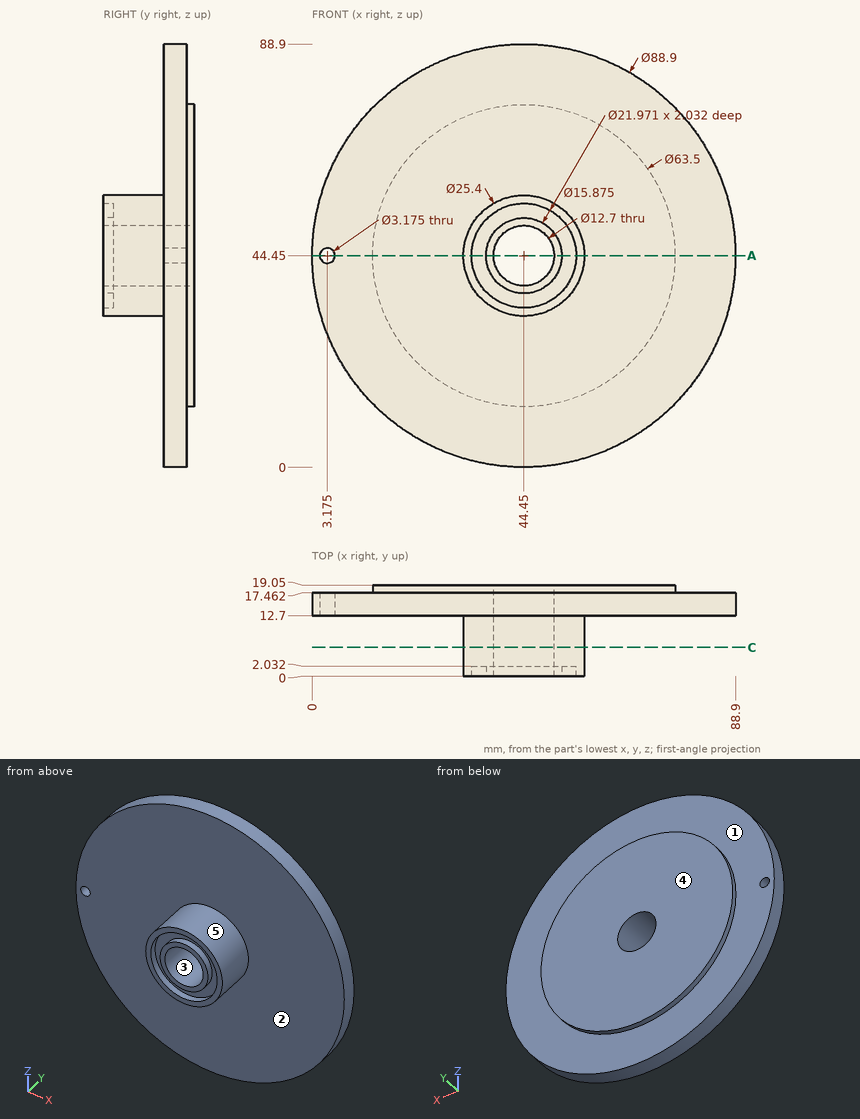
Could you check a few things on this drawing? It's one solid part, dimensions in mm from its lowest x, y, z. A direction names the side the tool comes from. Coordinates: 2 decimals unless noted, no trailing zeros. Order: outer loops, then holes, each group sorted by start corner. A loop starts at its lowest first (then second) coordinate and runs counter-clockwise, first axis right, second up. Notation, with made-up numbers: M 57,33 L 103,33 A24 cw 103,43 Z; hole C 46,-12.75 d10. An arc over 180 degrees is marked long. Answer as a JSON object with one key per item and string values. Group by question number.
(1) Suppose I cut it at A-A, the plane z = 44.45. State how many separate pieces and enclosed holes the cut face has.
(2) For pin 1 (7.5 mm diameter, centred on x = 44.45, z = 44.45, fed in from +Y); pin 2 (6 mm diameter, centred on x = 39, y = 2, fed in from -Z); pin 3 (5 mm diameter, centred on x = 3.175, z = 44.45, fed in from -Y), each with a flat end and sliding along its axis, tell me the tip position at first contact or that it passes through.
(3) I need wall thicknesses on probe 1 along Z at (x, y) = (44.45, 7.25); probe 2 along Y at (x, z) = (70, 61); probe 3 along Y at (x, z) = (81.5, 58.5). Which ranges of each line are inside material? Lowest first, please.
(4) Suppose I cut it at C-C, the plane y = 6. Please give me the cut outline in (x, z), then the cut area to 3 significant figures.
(5) Which directions (+Z, -Z, +X, -X, +Y, -Y) give clear straight access to the entire face, cutting with the end or side of a thin tool? Please do the marked faces 1 and 2.
(6) If we mould it in two halves opening along Z, with no side actions, what happens to the marked faces 3, 4 and 5? For each: released by +Z, released by -Z, zero draft, split by the parting line, or undercut.
Values found:
{
 "1": {"separate pieces": "3", "enclosed holes": "0"},
 "2": {"pin 1": "passes through", "pin 2": "stops at z = 31.99", "pin 3": "stops at y = 12.7"},
 "3": {"probe 1": "z = 31.75 to 38.1, 50.8 to 57.15", "probe 2": "y = 12.7 to 19.05", "probe 3": "y = 12.7 to 17.46"},
 "4": {"outline": "C 44.45,44.45 d25.4; hole C 44.45,44.45 d12.7", "area": "380 mm^2"},
 "5": {"face 1": "+Y", "face 2": "-Y"},
 "6": {"face 3": "undercut", "face 4": "zero draft", "face 5": "split by the parting line"}
}
